from build123d import *

# Parameters (mm, degrees)
SKETCH_1_R               = 27.5
EXTRUDE_1_DEPTH          = 10
SKETCH_2_R               = 10
EXTRUDE_2_DEPTH          = 3
SKETCH_3_R               = 2.75
CUT_EXTRUDE_1_DEPTH      = 30
PATTERN_CIRCULAR_1_COUNT = 4
SKETCH_4_R               = 5
CUT_EXTRUDE_2_DEPTH      = 10
PATTERN_CIRCULAR_2_COUNT = 4
SKETCH_5_W               = 66.473755295
SKETCH_5_H               = 48
CUT_EXTRUDE_3_DEPTH      = 3
CHAMFER_1_SIZE           = 1
CHAMFER_2_SIZE           = 1


with BuildPart() as part:
    # 草图1 → 凸台-拉伸1 (new, symmetric)
    with BuildSketch(Plane(origin=(0, 0, 0), x_dir=(0, 0, -1), z_dir=(1, 0, 0))):
        Circle(SKETCH_1_R)
    extrude(amount=EXTRUDE_1_DEPTH, both=True)

    # 草图2 → 凸台-拉伸2 (add)
    with BuildSketch(Plane(origin=(10, 0, 0), x_dir=(0, 0, -1), z_dir=(1, 0, 0))):
        Circle(SKETCH_2_R)
    extrude(amount=EXTRUDE_2_DEPTH)

    # 草图3 → 切除-拉伸1 (cut)
    with BuildSketch(Plane.ZY.offset(10)):
        with Locations((11.313708499, 11.313708499)):
            Circle(SKETCH_3_R)
    cut_extrude_1 = extrude(amount=-CUT_EXTRUDE_1_DEPTH, mode=Mode.SUBTRACT)

    # 阵列(圆周)1: 切除-拉伸1 ×4 about axis
    pattern_circular_1_axis = Axis((0, 0, 0), (1, 0, 0))
    for i in range(1, PATTERN_CIRCULAR_1_COUNT):
        add(cut_extrude_1.rotate(pattern_circular_1_axis, i * 360 / PATTERN_CIRCULAR_1_COUNT), mode=Mode.SUBTRACT)

    # 草图4 → 切除-拉伸2 (cut)
    with BuildSketch(Plane.ZY.offset(10)):
        with Locations((-11.313708499, 11.313708499)):
            Circle(SKETCH_4_R)
    cut_extrude_2 = extrude(amount=-CUT_EXTRUDE_2_DEPTH, mode=Mode.SUBTRACT)

    # 阵列(圆周)2: 切除-拉伸2 ×4 about axis
    pattern_circular_2_axis = Axis((0, 0, 0), (1, 0, 0))
    for i in range(1, PATTERN_CIRCULAR_2_COUNT):
        add(cut_extrude_2.rotate(pattern_circular_2_axis, i * 360 / PATTERN_CIRCULAR_2_COUNT), mode=Mode.SUBTRACT)

    # 草图5 → 切除-拉伸3 (cut)
    with BuildSketch(Plane.ZY.offset(10)):
        with Locations((4.248104101, 0)):
            Rectangle(SKETCH_5_W, SKETCH_5_H)
    extrude(amount=-CUT_EXTRUDE_3_DEPTH, mode=Mode.SUBTRACT)

    # 倒角1
    chamfer_1_edges = [part.edges().sort_by_distance(p)[0] for p in [
        (-10, 24, 0),
        (-10, -24, 0),
    ]]
    chamfer(chamfer_1_edges, length=CHAMFER_1_SIZE)

    # 倒角2
    chamfer_2_edges = [part.edges().sort_by_distance(p)[0] for p in [
        (10, 0, 27.5),
        (13, 0, 10),
    ]]
    chamfer(chamfer_2_edges, length=CHAMFER_2_SIZE)

    # 草图6 → M5 螺纹孔1 (revolve, cut)
    with BuildSketch(Plane(origin=(-7, -7.5, -20), x_dir=(0, 0, 1), z_dir=(0, 1, 0))):
        Polygon((0, 0), (0, 33.6618073), (2.1, 32.4), (2.1, 0), align=None)
    hole_wizard_m5_1 = revolve(axis=Axis((-13.35, -7.5, -20), (1, 0, 0)), mode=Mode.SUBTRACT)

    # 镜向1: M5 螺纹孔1 across plane
    add(hole_wizard_m5_1.mirror(Plane.ZX), mode=Mode.SUBTRACT)

    # 镜向2: M5 螺纹孔1 across plane
    add(hole_wizard_m5_1.mirror(Plane.XY), mode=Mode.SUBTRACT)

    # 镜向2 copy 1 sketch → 镜向2 copy 1 (revolve, cut)
    with BuildSketch(Plane(origin=(-7, 7.5, 20), x_dir=(0, 0, -1), z_dir=(0, -1, 0))):
        Polygon((0, 0), (0, 33.6618073), (2.1, 32.4), (2.1, 0), align=None)
    revolve(axis=Axis((-13.35, 7.5, 20), (1, 0, 0)), mode=Mode.SUBTRACT)


solid = part.part
Input: part model. Units: mm. Frame: model coordinates. A direction names the side the tool comes from. Coordinates: 2 decimals unless noted, no trailing zeros. Loops run counter-clockwise (first coordinate to the right, second up) from the corner with the lowest first, then second, coordinate; pieces in that order, holes last.
Q1. Contact query for flat-ended pins moving along their axis: pin 1 (6.5 mm diameter, centred on y = -7.5, z = -20, fed in from +X); pin 2 (6 mm diameter, centred on x = -3.5, y = -9.5, fed in from +Z); pin 3 (5.5 mm diameter, centred on y = -7.5, z = 20, fed in from -X); pin 4 (2.5 mm diameter, centred on y = 7.5, z = 20, fed in from -X). Output: stop coordinate, or through.
Q2. Draft query along Z for faces 4 (the face through (-10, -26, 0)), 5 (the face through (-0.367, -26.846, 5.961)), 6 (the face through (-3.549, -9.399, 6.695)). Return one class per face: +Z half, -Z half, draft (parallel to the pull), parting line (faces both ways), or undercut.
Q3. Material intervals for line 1 (Y direction, x = -0.5, z = 14); line 2 (Y direction, x = 8.75, z = -13.5); line 3 (Z direction, x = 7, y = 8.5), sorted ascending.
Q4. Cut plane A-A (z = 0). Output: boundary loops of the cut face in (x, y), then the cut area to 3 significant figures.
Q5. Set-up query: faces 1 (the face through (-8, -24, 0)), 2 (the face through (10, 0, -11)), 3 (the face through (-3.549, 6.695, 9.399)). Return all of +Z, -Z, +X, -X, +Y, -Y with unobstructed straight access to the full face (end or side cutting, diameter ignored); none if empty.
Q6. Cut plane B-B (y = 7.5). Give the number of separate pieces and of enclosed holes in the cut face, then the cut area to 3 significant figures.
Working result:
1. pin 1: stops at x = 10
1. pin 2: stops at z = 26.72
1. pin 3: stops at x = -7
1. pin 4: passes through
2. face 4: draft
2. face 5: parting line
2. face 6: undercut
3. line 1: y = -23.67 to -15.53, -7.1 to 7.1, 15.53 to 23.67
3. line 2: y = -23.96 to -12.98, -9.65 to 9.65, 12.98 to 23.96
3. line 3: z = -26.15 to -21.85, -18.15 to 18.15, 21.85 to 26.15
4. outline: (-10, -27.5) - (9, -27.5) - (10, -26.5) - (10, -10) - (12, -10) - (13, -9) - (13, 9) - (12, 10) - (10, 10) - (10, 26.5) - (9, 27.5) - (-10, 27.5) - (-10, 25) - (-9, 24) - (-7, 24) - (-7, -24) - (-9, -24) - (-10, -25) - close
4. area: 1,010 mm2
5. face 1: +Z, -Z, -X
5. face 2: +X
5. face 3: -X
6. separate pieces: 3
6. enclosed holes: 0
6. area: 703 mm2
